```python
from build123d import *

# Parameters (mm, degrees)
F1_DEPTH = 63.5
F0_W     = 25.4
F0_H     = 19.05
F2_DEPTH = 25.4
F3_DEPTH = 7.9375
F5_R     = 6.35


# Not quite as in the source:
# - a feature names something its author has since deleted; it is built from what else it names


with BuildPart() as f1:
    # F0 (on Front) → F1 (new body, symmetric)
    with BuildSketch(Plane.XZ):
        Polygon((-41.275, -9.525), (41.275, -9.525), (41.275, 9.525), (22.225, 9.525), (-41.275, 9.525), align=None)
    extrude(amount=F1_DEPTH, both=True)

    # F0 (on Front) → F2 (join, symmetric)
    with BuildSketch(Plane.XZ):
        with BuildLine():
            Line((22.225, 9.525), (41.275, 9.525))
            Line((41.275, 9.525), (41.275, 27.0002))
            ThreePointArc((41.275, 27.0002), (45.9246798487, 38.2255201513), (57.15, 42.8752))
            Line((57.15, 42.8752), (60.325, 42.8752))
            Line((60.325, 42.8752), (60.325, 61.9252))
            Line((60.325, 61.9252), (57.15, 61.9252))
            add(Edge.make_bspline(
                [(56.3025201656, 61.914916137), (56.5862693172, 61.9189290335), (56.8687741652, 61.9223540897), (57.15, 61.9252)],
                knots=[110.666674481, 110.666674481, 110.666674481, 110.666674481, 111.5045361635, 111.5045361635, 111.5045361635, 111.5045361635], degree=3))
            ThreePointArc((56.3025201656, 61.914916137), (32.156462253, 51.3944348905), (22.225, 27.0002))
            Line((22.225, 27.0002), (22.225, 9.525))
        make_face()
        with Locations((73.025, 52.4002)):
            Rectangle(F0_W, F0_H)
    extrude(amount=F2_DEPTH, both=True)

    # F0 (on Front) → F3 (join, symmetric)
    with BuildSketch(Plane.XZ):
        with BuildLine():
            add(Edge.make_bspline(
                [(-41.275, 9.525), (-40.3617250948, 50.5995517259), (18.8242875965, 61.3848836588), (56.3025201656, 61.914916137)],
                knots=[0, 0, 0, 0, 110.666674481, 110.666674481, 110.666674481, 110.666674481], degree=3))
            Line((-41.275, 9.525), (22.225, 9.525))
            Line((22.225, 9.525), (22.225, 27.0002))
            ThreePointArc((22.225, 27.0002), (32.156462253, 51.3944348905), (56.3025201656, 61.914916137))
        make_face()
    extrude(amount=F3_DEPTH, both=True)

    # F0 (on Front) → F4 (revolve)
    with BuildSketch(Plane.XZ):
        Polygon((85.725, 61.9252), (85.725, 42.8752), (85.725, 38.1), (111.125, 38.1), (111.125, 66.675), (85.725, 66.675), align=None)
    revolve(axis=Axis((85.725, 0, 52.3875), (0, 0, -1)))

    # F5
    f5_edges = [f1.edges().sort_by_distance(p)[0] for p in [
        (-41.275, -63.5, 0),
        (41.275, -63.5, 0),
        (41.275, 63.5, 0),
        (-41.275, 63.5, 0),
    ]]
    fillet(f5_edges, radius=F5_R)


solid = f1.part
```
Input: part model. Units: mm. Frame: model coordinates. A direction names the side the tool comes from. Give positions to 0.01 mm unless a question says otherwise; leave off trailing zeros. Loops run counter-clockwise (first coordinate to the right, second up) from the corner with the lowest first, then second, coordinate; pieces in that order, holes last. Notation, with made-up numbers: M 1,-31.5 L 36,-31.5 A21 ccw 36,6.5 Z; hole C -18.75,-8 d7. An arc over 180 degrees is marked long. Answer as CSV lines item,"result". Start each with the question number.
1. Pin query (flat end, axial travel): P1, Ø14, axis at y = -17.5, z = 20.5, coming from the -X side (3 decimals); P2, Ø3, axis at x = 16, z = 21.5, coming from the -Y side; P3, Ø5, axis at y = -6.5, z = 25, coming from the +X side. Return the tip coordinate at first contact, or that it passes through.
2. Section A-A on x = 66. Return loops of the section in (y, z) (3 decimals), plus the area to 3 significant figures.
3. Section C-C on x = 98.5. Return loops of the section in (y, z) (3 decimals), plus the area to 3 significant figures.
4. Pull-direction query (X, two-part tool) for faces 6 (the face through (-41.275, -1, 0)), 7 (the face through (1, -36, 9.525)), 8 (the face through (45.8, -0.4, 38.1)); classes: released by +X, released by -X, zero draft, split by the parting line, or undercut.
5. Section B-B on y = -30. Return loops of the section in (x, z) (3 decimals).
6. Line query: L1, parallel to Z at x = 26.5, y = -45 (3 decimals); L2, parallel to X at y = 47, z = 7.5 (3 decimals); L3, parallel to Y at x = 22, z = 33. Output: solid intervals per line, ascending.
7. Reachability of faces 1 (the face through (-3, -7.938, 30)), 2 (the face through (22.225, 17, 18)), 3 (the face through (46, 25.4, 42)), 4 (the face through (60, -2, 61.925)), 5 (the face through (86, 0, 38.1)) from +Z, -Z, +X, -X, +Y, -Y: full face, straight path, thin tool, end or side. Return the list, or none.
Computed values:
1,P1,"stops at x = 22.225"
1,P2,"stops at y = -7.94"
1,P3,"stops at x = 41.28"
2,outline,"M -25.4,42.875 L -16.003,42.875 L -16.003,38.1 L 16.003,38.1 L 16.003,42.875 L 25.4,42.875 L 25.4,61.925 L 16.003,61.925 L 16.003,66.675 L -16.003,66.675 L -16.003,61.925 L -25.4,61.925 Z"
2,area,"1,270 mm²"
3,outline,"M -21.954,38.1 L 21.954,38.1 L 21.954,66.675 L -21.954,66.675 Z"
3,area,"1,250 mm²"
4,face 6,"released by -X"
4,face 7,"zero draft"
4,face 8,"undercut"
5,outline,"M -41.275,-9.525 L 41.275,-9.525 L 41.275,9.525 L -41.275,9.525 Z"
6,L1,"z = -9.525 to 9.525"
6,L2,"x = -41.275 to 41.275"
6,L3,"y = -7.94 to 7.94"
7,face 1,"+Z, -X, -Y"
7,face 2,"+Z, -X, +Y"
7,face 3,"+Z, +X, -X, +Y"
7,face 4,"+Z, -X"
7,face 5,"-Z, +X, +Y, -Y"
